from build123d import *

# Parameters (mm, degrees)
F1_DEPTH = 1500
F4_DEPTH = 150


# Not quite as in the source:
# - the program builds the solid bodies; features that only make, move or delete a surface that nothing else refers to are left out


with BuildPart() as f1:
    # F0 (on Top) → F1 (new body)
    with BuildSketch(Plane.XY):
        with BuildLine():
            Line((-62.3253015232, -63.5), (62.3253015232, -63.5))
            ThreePointArc((62.3253015232, -63.5), (65.8608354292, -62.0355339059), (67.3253015232, -58.5))
            Line((67.3253015232, -58.5), (67.3253015232, 58.5))
            ThreePointArc((67.3253015232, 58.5), (65.8608354292, 62.0355339059), (62.3253015232, 63.5))
            Line((62.3253015232, 63.5), (-62.3253015232, 63.5))
            ThreePointArc((-62.3253015232, 63.5), (-65.8608354292, 62.0355339059), (-67.3253015232, 58.5))
            Line((-67.3253015232, 58.5), (-67.3253015232, -58.5))
            ThreePointArc((-67.3253015232, -58.5), (-65.8608354292, -62.0355339059), (-62.3253015232, -63.5))
        make_face()
        with BuildLine():
            Line((-57.8253015232, 59), (57.8253015232, 59))
            ThreePointArc((57.8253015232, 59), (61.3608354292, 57.5355339059), (62.8253015232, 54))
            Line((62.8253015232, 54), (62.8253015232, -54))
            ThreePointArc((62.8253015232, -54), (61.3608354292, -57.5355339059), (57.8253015232, -59))
            Line((57.8253015232, -59), (-57.8253015232, -59))
            ThreePointArc((-57.8253015232, -59), (-61.3608354292, -57.5355339059), (-62.8253015232, -54))
            Line((-62.8253015232, -54), (-62.8253015232, 54))
            ThreePointArc((-62.8253015232, 54), (-61.3608354292, 57.5355339059), (-57.8253015232, 59))
        make_face(mode=Mode.SUBTRACT)
    extrude(amount=F1_DEPTH)

    # F2 (on face) → F4 (cut)
    with BuildSketch(Plane.YZ.offset(67.3253015232)):
        with BuildLine():
            ThreePointArc((-25.5, 1304), (-24.0355339059, 1300.4644660941), (-20.5, 1299))
            Line((-20.5, 1299), (20.5, 1299))
            ThreePointArc((20.5, 1299), (24.0355339059, 1300.4644660941), (25.5, 1304))
            Line((25.5, 1304), (25.5, 1445))
            ThreePointArc((25.5, 1445), (24.0355339059, 1448.5355339059), (20.5, 1450))
            Line((20.5, 1450), (-20.5, 1450))
            ThreePointArc((-20.5, 1450), (-24.0355339059, 1448.5355339059), (-25.5, 1445))
            Line((-25.5, 1445), (-25.5, 1304))
        make_face()
        with BuildLine():
            ThreePointArc((-25.5, 893), (-24.0355339059, 889.4644660941), (-20.5, 888))
            Line((-20.5, 888), (20.5, 888))
            ThreePointArc((20.5, 888), (24.0355339059, 889.4644660941), (25.5, 893))
            Line((25.5, 893), (25.5, 1034))
            ThreePointArc((25.5, 1034), (24.0355339059, 1037.5355339059), (20.5, 1039))
            Line((20.5, 1039), (-20.5, 1039))
            ThreePointArc((-20.5, 1039), (-24.0355339059, 1037.5355339059), (-25.5, 1034))
            Line((-25.5, 1034), (-25.5, 893))
        make_face()
        with BuildLine():
            ThreePointArc((-25.5, 482), (-24.0355339059, 478.4644660941), (-20.5, 477))
            Line((-20.5, 477), (20.5, 477))
            ThreePointArc((20.5, 477), (24.0355339059, 478.4644660941), (25.5, 482))
            Line((25.5, 482), (25.5, 623))
            ThreePointArc((25.5, 623), (24.0355339059, 626.5355339059), (20.5, 628))
            Line((20.5, 628), (-20.5, 628))
            ThreePointArc((-20.5, 628), (-24.0355339059, 626.5355339059), (-25.5, 623))
            Line((-25.5, 623), (-25.5, 482))
        make_face()
    extrude(amount=-F4_DEPTH, mode=Mode.SUBTRACT)


solid = f1.part
The listing builds one solid part. Answer for the finished solid, in the listing's coordinates (mm). A direction names the side the tool comes from. Give positions to 0.01 mm unless a question says otherwise; leave off trailing zeros. Loops run counter-clockwise (first coordinate to the right, second up) from the corner with the lowest first, then second, coordinate; pieces in that order, holes last. Notation, with made-up numbers: (34, 70) - (90, 70) arc R18 cw to (90, 105) - close; hole circle Ø11 at (-39.5, -5). An arc over 180 degrees is marked (long way). Answer as a JSON object with one key per item and string values.
1. A cutting plane is placed at B-B (x = -1.5). Write down the section's boundary in (y, z), then the cut area to 3 significant figures.
Determined:
{"outline": "(-63.5, 0) - (-59, 0) - (-59, 1500) - (-63.5, 1500) - close; (59, 0) - (63.5, 0) - (63.5, 1500) - (59, 1500) - close", "area": "13,500 mm²"}
2. A cutting plane is placed at C-C (y = 4). Give the number of separate pieces and of enclosed holes in the cut face, then the cut area to 3 significant figures.
Determined:
{"separate pieces": "8", "enclosed holes": "0", "area": "9,420 mm²"}
3. A cutting plane is placed at A-A (z = 569). Write down the section's boundary in (x, y), then the cut area to 3 significant figures.
Determined:
{"outline": "(-67.33, -58.5) arc R5 ccw to (-62.33, -63.5) - (62.33, -63.5) arc R5 ccw to (67.33, -58.5) - (67.33, -25.5) - (62.83, -25.5) - (62.83, -54) arc R5 cw to (57.83, -59) - (-57.83, -59) arc R5 cw to (-62.83, -54) - (-62.83, -25.5) - (-67.33, -25.5) - close; (-67.33, 25.5) - (-62.83, 25.5) - (-62.83, 54) arc R5 cw to (-57.83, 59) - (57.83, 59) arc R5 cw to (62.83, 54) - (62.83, 25.5) - (67.33, 25.5) - (67.33, 58.5) arc R5 ccw to (62.33, 63.5) - (-62.33, 63.5) arc R5 ccw to (-67.33, 58.5) - close", "area": "1,810 mm²"}
4. Flat-ended cylindrical pins translate along their axes: pin 1 Ø5 at (x, z) = (-65, 1376) entering from +Y; pin 2 Ø5 at (x, z) = (66, 1380) entering from +Y; pin 3 Ø3.5 at (x, y) = (65, -2) entering from -Z; pin 4 Ø1.3 at (x, z) = (66, 518.5) entering from -Y. Find the tip coordinate at first contact, or state that the pin passes through.
Determined:
{"pin 1": "y = 63.5", "pin 2": "y = 63.36", "pin 3": "z = 0", "pin 4": "y = -62.48"}
5. Find the intervals of material crossed by L1, parallel to Y at x = 51, z = 684; L2, parallel to X at y = -45, z = 1405.5, in increasing order. Write a range as [from, to].
Determined:
{"L1": "[-63.5, -59], [59, 63.5]", "L2": "[-67.33, -62.83], [62.83, 67.33]"}
6. For a pull along Y with two mould halves and no side action, classify faces 1 (the flat face through (1, -59, 740)), 2 (the flat face through (1, 63.5, 740)), 3 (the flat face through (-67.325, 1, 740)) as pulls with the +Y half, pulls with the -Y half, needs draft (parallel to the pull), parting line crosses it, or undercut.
Determined:
{"face 1": "undercut", "face 2": "pulls with the +Y half", "face 3": "needs draft"}
7. For faces 4 (the flat face through (-62.825, -1, 740)), 5 (the flat face through (67.325, -1, 740)), determine the directions among +Z, -Z, +X, -X, +Y, -Y from which every point of the face is accessible in a straight line to the end or side of a thin tool.
Determined:
{"face 4": "+Z, -Z", "face 5": "+Z, -Z, +X, +Y, -Y"}
